Read the model definition and answer for the solid it produces. Units are mm, in the model's axes. A direction names the side the tool comes from. Coordinates: 2 decimals unless noted, no trailing zeros. Order: outer loops, then holes, each group sorted by start corner. A loop starts at its lowest first (then second) coordinate and runs counter-clockwise, first axis right, second up. Notation, with made-up numbers: M 68,23.25 L 101,23.25 A31 cw 101,56.25 Z; hole C 51.25,-0.75 d5. An arc over 180 degrees is marked long. Write each question's results on one line, items separated by ' | '.
```python
from build123d import *

# Parameters (mm, degrees)
F2_SIZE  = 10
F4_DEPTH = 1000


with BuildPart() as f1:
    # F0 (on Front) → F1 (revolve)
    with BuildSketch(Plane.XZ):
        Polygon((0, 200), (0, 0), (252.01218, 0), (252.01218, 73.99391), align=None)
    revolve(axis=Axis((191.066653, 0, 0), (1, 0, 0)))

    # F2
    f2_edges = [f1.edges().sort_by_distance(p)[0] for p in [
        (252.01218, 0, -73.99391),
    ]]
    chamfer(f2_edges, length=F2_SIZE)

    # F3 (on face) → F4 (cut)
    with BuildSketch(Plane(origin=(0, 0, 0), x_dir=(0, -1, 0), z_dir=(-1, 0, 0))):
        with BuildLine():
            Line((-15, 175.000831), (0, 175.000831))
            Line((0, 175.000831), (15, 175.000831))
            Line((15, 175.000831), (23.590783, 198.603814))
            ThreePointArc((23.590783, 198.603814), (0, 200), (-23.590783, 198.603814))
            Line((-23.590783, 198.603814), (-15, 175.000831))
        make_face()
    extrude(amount=-F4_DEPTH, mode=Mode.SUBTRACT)


solid = f1.part
```
(1) The part is cut by section C-C, the plane z = 0. Write down the section's boundary in (x, y), then the cut area to 3 significant figures.
Conclusion:
outline: M 0,-200 L 243.07,-78.47 L 252.01,-63.99 L 252.01,63.99 L 243.07,78.47 L 0,200 Z | area: 69,000 mm²
(2) For faces 1 (the flat face through (18.6, 18.4, 184.34)), 2 (the flat face through (252.012, -1, 1)), determine the directions among +Z, -Z, +X, -X, +Y, -Y from which every point of the face is accessible in a straight line to the end or side of a thin tool.
Conclusion:
face 1: +Z, +X, -X | face 2: +Z, -Z, +X, +Y, -Y
(3) Given pin 1 (6 mm diameter, centred on x = 152.5, y = 5.5, fed in from +Z); pin 2 (5 mm diameter, centred on x = 153, z = 6, fed in from +Y); pin 3 (5 mm diameter, centred on y = 144, z = -116.5, fed in from +X), each flat-ended and moving along its own axis, determine where each tip first touches the part or whether it passes through.
Conclusion:
pin 1: z = 125.13 | pin 2: y = 124.61 | pin 3: x = 34.55
(4) The mould has two halves that part along Y. Classify faces 3 (the flat face through (0, -3, -3)), 4 (the conical face through (251.45, 63.36, -14.07)), 5 (the flat face through (25, 0, 175.001)): pulls with the +Y half, pulls with the -Y half, needs draft (parallel to the pull), parting line crosses it, or undercut.
Conclusion:
face 3: needs draft | face 4: parting line crosses it | face 5: undercut
(5) The part is cut by section D-D, the plane x = 199.5. Write down the section's boundary in (y, z), then the cut area to 3 significant figures.
Conclusion:
outline: C 0,0 d200.5 | area: 31,600 mm²
(6) The part is cut by section B-B, the plane x = 136.5. Write down the section's boundary in (y, z), then the cut area to 3 significant figures.
Conclusion:
outline: C 0,0 d263.5 | area: 54,500 mm²
(7) Straight lines are drawn through the part: line 1 (Y direction, x = 204, z = -70); line 2 (X direction, y = -65, z = 176); line 3 (Y direction, x = 60, z = 95). For each, find the intervals that lie inside material, in ascending order.
Conclusion:
line 1: -68.59 to 68.59 | line 2: 0 to 24.76 | line 3: -140.98 to 140.98
(8) The part is cut by section A-A, the plane y = 0. Write down the section's boundary in (x, z).
Conclusion:
outline: M 0,-200 L 243.07,-78.47 L 252.01,-63.99 L 252.01,63.99 L 243.07,78.47 L 50,175 L 0,175 Z
